from build123d import *

# Parameters (mm, degrees)
PAD030_DEPTH         = 1
SKETCH054_R          = 3.5
PAD031_DEPTH         = 2.5
PAD032_DEPTH         = 5
SKETCH056_R          = 1.8
POCKET018_DEPTH      = 1.501
POCKET018_DEPTH_BACK = 8.001
CHAMFER005_SIZE      = 1
FILLET001_R          = 6
CHAMFER006_SIZE      = 0.3


with BuildPart() as part:
    # Sketch053 → Pad030 (new body)
    with BuildSketch(Plane.YZ.offset(45.5)):
        with BuildLine():
            ThreePointArc((40, 0), (35.4804333271, 18.4699445294), (22.943057454, 32.7660817716))
            Line((14.3394109088, 20.4788011072), (22.943057454, 32.7660817716))
            ThreePointArc((25, 0), (22.1752708295, 11.5437153309), (14.3394109088, 20.4788011072))
            Line((25, -5), (25, 0))
            Line((40, -5), (25, -5))
            Line((40, 0), (40, -5))
        make_face()
    extrude(amount=PAD030_DEPTH)

    # Sketch054 → Pad031 (join)
    with BuildSketch(Plane.YZ.offset(45.5)):
        with Locations((22.9809703886, 22.9809703886)):
            Circle(SKETCH054_R)
    extrude(amount=-PAD031_DEPTH)

    # Sketch055 → Pad032 (join)
    with BuildSketch(Plane.XY):
        Polygon((39, 39), (37, 39), (37, 26), (39, 26), (42.5, 28), (45.5, 28), (45.5, 37), (42.5, 37), align=None)
    extrude(amount=-PAD032_DEPTH)

    # Sketch056 → Pocket018 (cut, two sides)
    with BuildSketch(Plane.YZ.offset(45)) as pocket018_sk:
        with Locations((22.9809703886, 22.9809703886)):
            Circle(SKETCH056_R)
    extrude(amount=POCKET018_DEPTH, mode=Mode.SUBTRACT)
    extrude(pocket018_sk.sketch, amount=-POCKET018_DEPTH_BACK, mode=Mode.SUBTRACT)

    # Chamfer005
    chamfer005_edges = [part.edges().sort_by_distance(p)[0] for p in [
        (43, 21.18097, 22.98097),
    ]]
    chamfer(chamfer005_edges, length=CHAMFER005_SIZE)

    # Fillet001
    fillet001_edges = [part.edges().sort_by_distance(p)[0] for p in [
        (46, 14.339411, 20.478801),
        (46, 22.943057, 32.766082),
    ]]
    fillet(fillet001_edges, radius=FILLET001_R)

    # Chamfer006
    chamfer006_edges = [part.edges().sort_by_distance(p)[0] for p in [
        (43, 19.48097, 22.98097),
    ]]
    chamfer(chamfer006_edges, length=CHAMFER006_SIZE)


solid = part.part
The listing builds one solid part. Answer for the finished solid, in the listing's coordinates (mm). A direction names the side the tool comes from. Coordinates: 2 decimals unless noted, no trailing zeros. Loops run counter-clockwise (first coordinate to the right, second up) from the corner with the lowest first, then second, coordinate; pieces in that order, holes last.
1) Flat-ended cylindrical pins translate along their axes: pin 1 Ø0.9 at (x, z) = (43.5, -2.5) entering from +Y; pin 2 Ø12 at (y, z) = (33, 9.5) entering from -X; pin 3 Ø1.9 at (y, z) = (21.5, 22.5) entering from -X; pin 4 Ø2 at (y, z) = (22.98, 22.98) entering from -X. Find the tip coordinate at first contact, or state that the pin passes through.
2) Find the intervals of material crossed by L1, parallel to Z at x = 44.75, y = 23; L2, parallel to Z at x = 37.5, y = 33.75; L3, parallel to Y at x = 46, z = 0, in increasing order.
3) Find section B-B on z = -2. Write down the section's boundary in (x, y), then the cut area to 4 significant figures.
4) Find section A-A on y = 27.5. Write down the section's boundary in (x, z) (3 decimals).
5) Find section C-C on x = 38. Write down the section's boundary in (y, z), then the cut area to 3 significant figures.
6) Find section D-D on y = 38.25. Write down the section's boundary in (x, z).
7) Determine the mould class of faces 5 (the face through (40.73, 26.99, -2.46)), 6 (the face through (45.99, 37.06, 15.05)), 7 (the face through (46.5, 28, 13)) for opening direction X: pulls with the +X half, pulls with the -X half, needs draft (parallel to the pull), parting line crosses it, or undercut.
8) A tool of negligible diameter and unlimited length cuts with its end or side. For faces 1 (the face through (41, 33, 0)), 2 (the face through (38, 39, -2)), 3 (the face through (46, 25, -3)), 4 (the face through (44, 37, -2)), from which of +Z, -Z, +X, -X, +Y, -Y can it reach the whole face along a straight path? Write none if from no direction.
Values:
1. pin 1: stops at y = 37
1. pin 2: stops at x = 45.5
1. pin 3: stops at x = 43.29
1. pin 4: passes through
2. L1: z = 19.48 to 21.18, 24.78 to 26.48
2. L2: z = -5 to 0
2. L3: y = 25 to 40
3. outline: (37, 26) - (39, 26) - (42.5, 28) - (45.5, 28) - (45.5, 25) - (46.5, 25) - (46.5, 40) - (45.5, 40) - (45.5, 37) - (42.5, 37) - (39, 39) - (37, 39) - close
3. area: 106.5 mm2
4. outline: (37, -5) - (41.625, -5) - (41.625, 0) - (37, 0) - close; (45.5, -5) - (46.5, -5) - (46.5, 28.923) - (45.5, 28.923) - close
5. outline: (26, -5) - (39, -5) - (39, 0) - (26, 0) - close
5. area: 65.0 mm2
6. outline: (37, -5) - (40.31, -5) - (40.31, 0) - (37, 0) - close; (45.5, -5) - (46.5, -5) - (46.5, 11.7) - (45.5, 11.7) - close
7. face 5: undercut
7. face 6: needs draft
7. face 7: pulls with the +X half
8. face 1: +Z, -X, +Y, -Y
8. face 2: +Z, -Z, -X, +Y
8. face 3: -Z, +X, -X, -Y
8. face 4: +Z, -Z, +Y
